Geometry check sheet. Reference: the model listing, model coordinates, mm. Face numbers are marked on the shaded views. A direction names the side the tool comes from. Coordinates: 2 decimals unless noted, no trailing zeros. Write each loop counter-clockwise with the first axis right and the second up, starting at its lowest first coordinate (ties: lowest second). Pieces come first, ordered by that corner, then holes. Notation, with made-up numbers: M -10.5,55 L 16.5,55 A7 ccw 16.5,59 Z; hole C 73,52.25 d8. An arc over 180 degrees is marked long. Put each result on its own line as item: value. Start each with the question number.
1) Cross-section at B-B on y = 8.5. Record the cut outline in (x, z).
2) Cross-section at C-C on z = -25.75. Record the cut outline in (x, y).
3) Gauge pin test, flat ends, axial feed: pin 1 (6 mm diameter, centred on x = 5.5, z = 13, fed in from -Y); pin 2 (5 mm diameter, centred on y = 9, z = -13.5, fed in from +X); pin 3 (1.5 mm diameter, centred on x = 9, z = 15, fed in from +Y). Record the tip position at first contact, or that the pin passes through.
4) Cross-section at D-D on x = 2. Record the cut outline in (y, z).
5) Scan lines: line 1 along X through (y, z) = (2.1, 25.75); line 2 along Y through (x, z) = (0.75, -15.5); line 3 along X through (y, z) = (11.75, -3.5). Record each from-to range of solid material in increasing order.
6) Cross-section at A-A on x = 11.05. Record the cut outline in (y, z).
7) Set-up check for the marked faces 1 and 2: record each of +Z, -Z, +X, -X, +Y, -Y from which the full face is reachable in a straight line by a thin tool's end or side.
from build123d import *

# Parameters (mm, degrees)
EXTRUDE_THIN1_DEPTH = 32.5
CUT_EXTRUDE2_REACH  = 44.214
SKETCH4_R           = 2
SKETCH3_R           = 2.5
CUT_EXTRUDE1_DEPTH  = 3


with BuildPart() as part:
    # Sketch1 → Extrude-Thin1 (new, symmetric)
    with BuildSketch(Plane.XY):
        Polygon((19.05, 0), (0, 0), (0, 19.05), (3, 19.05), (3, 3), (19.05, 3), align=None)
    extrude(amount=EXTRUDE_THIN1_DEPTH, both=True)

    # Sketch4 → Cut-Extrude2 (cut, up to next)
    with BuildSketch(Plane.ZY, mode=Mode.PRIVATE) as cut_extrude2_sk1:
        with Locations((-15.5, 8.5)):
            Circle(SKETCH4_R)
    cut_extrude2_tool1 = extrude(cut_extrude2_sk1.sketch, amount=-CUT_EXTRUDE2_REACH, mode=Mode.PRIVATE) & part.part
    # Sketch4 → Cut-Extrude2 (cut, up to next)
    with BuildSketch(Plane.ZY, mode=Mode.PRIVATE) as cut_extrude2_sk2:
        with Locations((15.5, 8.5)):
            Circle(SKETCH4_R)
    cut_extrude2_tool2 = extrude(cut_extrude2_sk2.sketch, amount=-CUT_EXTRUDE2_REACH, mode=Mode.PRIVATE) & part.part
    add(cut_extrude2_tool1.solids().sort_by_distance((0, 8.5, -15.5))[0], mode=Mode.SUBTRACT)
    add(cut_extrude2_tool2.solids().sort_by_distance((0, 8.5, 15.5))[0], mode=Mode.SUBTRACT)

    # Sketch3 → Cut-Extrude1 (cut)
    with BuildSketch(Plane.XZ):
        with Locations(Location((11.05, -25.75, 0), (0, 0, 270))):
            Circle(SKETCH3_R)
        with Locations(Location((11.05, 25.75, 0), (0, 0, 270))):
            Circle(SKETCH3_R)
    extrude(amount=-CUT_EXTRUDE1_DEPTH, mode=Mode.SUBTRACT)


solid = part.part
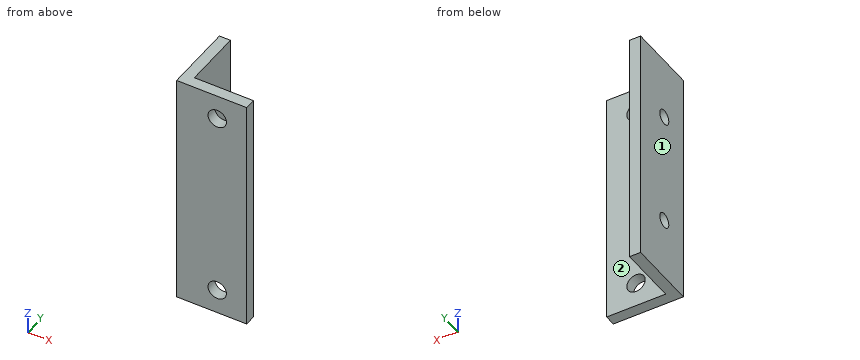
Answer key:
1. outline: M 0,-32.5 L 3,-32.5 L 3,-17.5 L 0,-17.5 Z; M 0,-13.5 L 3,-13.5 L 3,13.5 L 0,13.5 Z; M 0,17.5 L 3,17.5 L 3,32.5 L 0,32.5 Z
2. outline: M 0,0 L 8.55,0 L 8.55,3 L 3,3 L 3,19.05 L 0,19.05 Z; M 13.55,0 L 19.05,0 L 19.05,3 L 13.55,3 Z
3. pin 1: stops at y = 0
3. pin 2: stops at x = 3
3. pin 3: stops at y = 3
4. outline: M 0,-32.5 L 19.05,-32.5 L 19.05,32.5 L 0,32.5 Z; hole C 8.5,-15.5 d4; hole C 8.5,15.5 d4
5. line 1: x = 0 to 8.55, 13.55 to 19.05
5. line 2: y = 0 to 6.5, 10.5 to 19.05
5. line 3: x = 0 to 3
6. outline: M 0,-32.5 L 3,-32.5 L 3,-28.25 L 0,-28.25 Z; M 0,-23.25 L 3,-23.25 L 3,23.25 L 0,23.25 Z; M 0,28.25 L 3,28.25 L 3,32.5 L 0,32.5 Z
7. face 1: +Z, -Z, -X, +Y, -Y
7. face 2: +Z, -Z, +X, +Y
